Check sheet for the modelled part. Datum: model origin and axes. Units: mm. Face numbers are marked on the shaded views. A direction names the side the tool comes from. Give positions to 0.01 mm unless a question says otherwise; leave off trailing zeros. Order: outer loops, then holes, each group sorted by start corner. A loop starts at its lowest first (then second) coordinate and runs counter-clockwise, first axis right, second up.
Item 1: Gauge pin test, flat ends, axial feed: P1, Ø3, axis at y = 3, z = -5.5, coming from the +X side; P2, Ø5, axis at y = 34.5, z = -3.5, coming from the +X side; P3, Ø5, axis at y = 43, z = -33, coming from the -X side; P4, Ø3, axis at x = 11, z = -43.5, coming from the -Y side. Record the tip position at first contact, or that the pin passes through.
Item 2: Sectioned sample at A-A on y = 14. Record the boundary of the cut face in (x, z), and give its area (3 significant figures).
Item 3: Access from +Z, -Z, +X, -X, +Y, -Y to the whole of each face (thin tool, end or side, straight path). Record for the marked faces 1, 2, 3, 4 and 5.
Item 4: Sectioned sample at C-C on x = 39. Record the boundary of the cut face in (y, z).
Item 5: Sectioned sample at D-D on y = 6. Record the boundary of the cut face in (x, z), and give its area (3 significant figures).
Item 6: Material ranges on line 1 along Y through (x, z) = (5.5, -32); line 2 along X through (y, z) = (43.5, -42.5); line 3 along Z through (x, y) = (25.5, 42), recorded low to high.
Item 7: Sectioned sample at B-B on z = -27. Record the boundary of the cut face in (x, y), and give its area (3 significant figures).
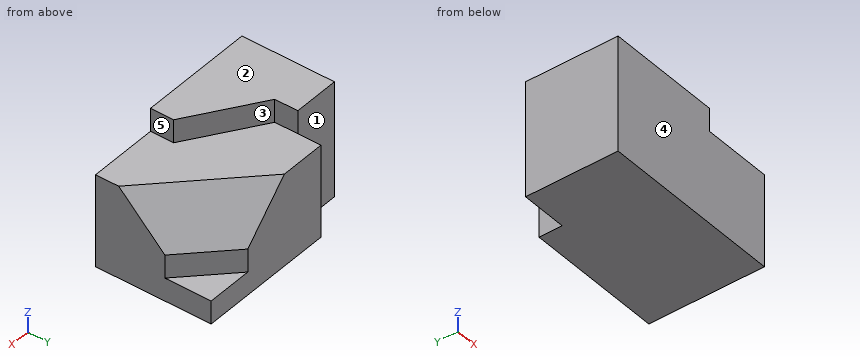
from build123d import *

# Parameters (mm, degrees)
SKETCH2_W           = 80
SKETCH2_H           = 50
BOSS_EXTRUDE1_DEPTH = 10
SKETCH3_W           = 30
SKETCH3_H           = 10
CUT_EXTRUDE1_DEPTH  = 10
SKETCH4_W           = 60
SKETCH4_H           = 40
BOSS_EXTRUDE2_DEPTH = 40
BOSS_EXTRUDE3_DEPTH = 50
CUT_EXTRUDE2_DEPTH  = 50
CUT_EXTRUDE3_DEPTH  = 50


with BuildPart() as part:
    # Sketch2 → Boss-Extrude1 (new body)
    with BuildSketch(Plane(origin=(0, 0, 0), x_dir=(1, 0, 0), z_dir=(0, 1, 0))):
        with Locations((40, 25)):
            Rectangle(SKETCH2_W, SKETCH2_H)
    extrude(amount=BOSS_EXTRUDE1_DEPTH)

    # Sketch3 → Cut-Extrude1 (cut)
    with BuildSketch(Plane(origin=(0, 10, 0), x_dir=(1, 0, 0), z_dir=(0, 1, 0))):
        with Locations((65, 5)):
            Rectangle(SKETCH3_W, SKETCH3_H)
    extrude(amount=-CUT_EXTRUDE1_DEPTH, mode=Mode.SUBTRACT)

    # Sketch4 → Boss-Extrude2 (add)
    with BuildSketch(Plane(origin=(0, 10, 0), x_dir=(1, 0, 0), z_dir=(0, 1, 0))):
        with Locations((50, 30)):
            Rectangle(SKETCH4_W, SKETCH4_H)
    extrude(amount=BOSS_EXTRUDE2_DEPTH)

    # Sketch5 → Boss-Extrude3 (add)
    with BuildSketch(Plane.XY):
        Polygon((20, 30), (50, 10), (0, 10), (0, 40), (20, 40), align=None)
    extrude(amount=-BOSS_EXTRUDE3_DEPTH)

    # Sketch6 → Cut-Extrude2 (cut)
    with BuildSketch(Plane.XY.offset(-40)):
        Polygon((60, 50), (80, 30), (80, 50), align=None)
    extrude(amount=CUT_EXTRUDE2_DEPTH, mode=Mode.SUBTRACT)

    # Sketch9 → Cut-Extrude3 (cut)
    with BuildSketch(Plane(origin=(26.666666667, 26.666666667, 26.666666667), x_dir=(-0.816496581, 0.40824829, 0.40824829), z_dir=(-0.577350269, -0.577350269, -0.577350269))):
        Polygon((-16.329931619, 42.426406871), (-40.824829046, 56.568542495), (-65.319726474, 42.426406871), (-65.319726474, 14.142135624), align=None)
    extrude(amount=-CUT_EXTRUDE3_DEPTH, mode=Mode.SUBTRACT)


solid = part.part
Report:
1. P1: stops at x = 50
1. P2: stops at x = 20
1. P3: stops at x = 20
1. P4: stops at y = 0
2. outline: (0, -50) - (80, -50) - (80, -14) - (76, -10) - (44, -10) - (44, 0) - (0, 0) - close
2. area: 3,630 mm2
3. face 1: +Z, -Z, -X, +Y
3. face 2: +Z, +X, -X, +Y, -Y
3. face 3: +Z, +X, +Y
3. face 4: +Z, -Z, +X, -X, -Y
3. face 5: +Z, +X, +Y, -Y
4. outline: (0, -50) - (50, -50) - (50, -10) - (17.33, -10) - (17.33, 0) - (0, 0) - close
5. outline: (0, -50) - (80, -50) - (80, -10) - (50, -10) - (50, 0) - (0, 0) - close
5. area: 3,700 mm2
6. line 1: y = 0 to 40
6. line 2: x = 20 to 80
6. line 3: z = -50 to -10
7. outline: (0, 0) - (80, 0) - (80, 27) - (57, 50) - (20, 50) - (20, 40) - (0, 40) - close
7. area: 3,540 mm2
